The listing builds one solid part. Answer for the finished solid, in the listing's coordinates (mm). Face numbers are marked on the shaded views. A direction names the side the tool comes from. Give positions to 0.01 mm unless a question says otherwise; leave off trailing zeros. Order: outer loops, then holes, each group sorted by start corner. A loop starts at its lowest first (then second) coordinate and runs counter-clockwise, first axis right, second up.
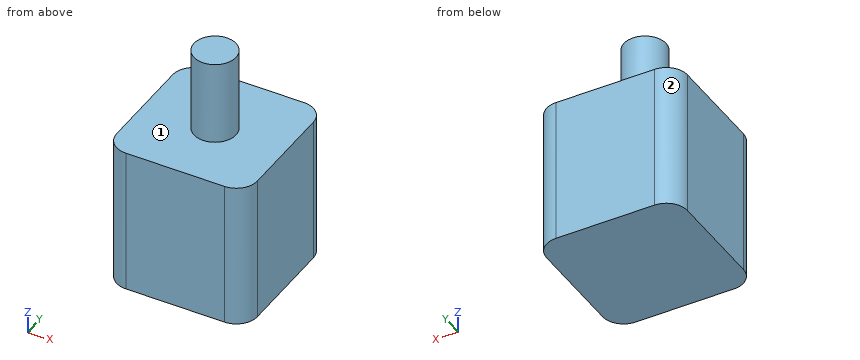
```python
from build123d import *

# Parameters (mm, degrees)
SKETCH1_W           = 42.545
SKETCH1_H           = 42.545
BOSS_EXTRUDE1_DEPTH = 44.45
FILLET2_R           = 6.35
SKETCH2_R           = 6.35
BOSS_EXTRUDE2_DEPTH = 69.85


with BuildPart() as part:
    # Sketch1 → Boss-Extrude1 (new body)
    with BuildSketch(Plane.XY):
        with Locations((21.2725, 21.2725)):
            Rectangle(SKETCH1_W, SKETCH1_H)
    extrude(amount=BOSS_EXTRUDE1_DEPTH)

    # Fillet2
    fillet2_edges = [part.edges().sort_by_distance(p)[0] for p in [
        (0, 42.545, 22.225),
        (42.545, 42.545, 22.225),
        (42.545, 0, 22.225),
        (0, 0, 22.225),
    ]]
    fillet(fillet2_edges, radius=FILLET2_R)

    # Sketch2 → Boss-Extrude2 (add)
    with BuildSketch(Plane(origin=(0, 0, 0), x_dir=(-1, 0, 0), z_dir=(0, 0, -1))):
        with Locations((-21.2725, 21.2725)):
            Circle(SKETCH2_R)
    extrude(amount=-BOSS_EXTRUDE2_DEPTH)


solid = part.part
```
1) Straight lines are drawn through the part: probe 1 along Z at (x, y) = (27, 35); probe 2 along X at (y, z) = (6, 11); probe 3 along Y at (x, z) = (18, 52). For each, find the intervals that lie inside material, in ascending order.
Geometry says:
probe 1: z = 0 to 44.45
probe 2: x = 0.01 to 42.54
probe 3: y = 15.83 to 26.71
2) Given P1, Ø4, axis at x = 6.5, y = 15.5, coming from the +Z side; P2, Ø4, axis at y = 25.5, z = 52.5, coming from the +X side, each flat-ended and moving along its own axis, determine where each tip first touches the part or whether it passes through.
Geometry says:
P1: stops at z = 44.45
P2: stops at x = 27.22
3) A tool of negligible diameter and unlimited length cuts with its end or side. For the marked faces 1 and 2, from which of +Z, -Z, +X, -X, +Y, -Y can it reach the whole face along a straight path? Write none if from no direction.
Geometry says:
face 1: +Z
face 2: +Z, -Z, -X, +Y
4) Find section A-A (z = 32). Write down the section's boundary in (x, y) (3 decimals), then the cut area to 3 significant figures.
Geometry says:
outline: (0, 6.35) arc R6.35 ccw to (6.35, 0) - (36.195, 0) arc R6.35 ccw to (42.545, 6.35) - (42.545, 36.195) arc R6.35 ccw to (36.195, 42.545) - (6.35, 42.545) arc R6.35 ccw to (0, 36.195) - close
area: 1,780 mm2
5) Find section B-B (x = 22.5). Write down the section's boundary in (y, z) (3 decimals), then the cut area to 3 significant figures.
Geometry says:
outline: (0, 0) - (42.545, 0) - (42.545, 44.45) - (27.503, 44.45) - (27.503, 69.85) - (15.042, 69.85) - (15.042, 44.45) - (0, 44.45) - close
area: 2,210 mm2
6) Find section C-C (y = 13). Write down the section's boundary in (x, z) (3 decimals).
Geometry says:
outline: (0, 0) - (42.545, 0) - (42.545, 44.45) - (0, 44.45) - close
7) Find section D-D (z = 45.5). Write down the section's boundary in (x, y).
Geometry says:
outline: circle Ø12.7 at (21.27, 21.27)
